Could you check a few things on this model? Use its own coordinates, in mm. A direction names the side the tool comes from. Round coordinates to 2 decimals unless told otherwise and drop trailing zeros. Loops run counter-clockwise (first coordinate to the right, second up) from the corner with the lowest first, then second, coordinate; pieces in that order, holes last. Notation, with made-up numbers: (-37.5, 51.5) -> (5.5, 51.5) arc R16 cw to (5.5, 73.5) -> close; hole circle Ø3 at (38, 48.5). An arc over 180 degrees is marked (long way). Write each question's results on one line, items separated by ' | '. Start each with the question number.
1) We'd pull the mould along Y, two halves only. Please class faces 1 (the flat face through (0, 3, 0)), 2 (the cylindrical face through (-0.33, -7.493, 3.944)), 3 (the flat face through (1.97, -3.48, 5.54)): pulls with the +Y half, pulls with the -Y half, needs draft (parallel to the pull), parting line crosses it, or undercut.
2) Imagine slicing it at C-C, the plane x = 1. List the corners of the cut face in (y, z) for me.
3) Imagine slicing it at A-A, the plane y = 0. List the corners of the cut face in (x, z) for me, plus the area to 3 significant figures.
4) Imagine slicing it at B-B, the plane z = 4.5. List the corners of the cut face in (x, y) for me, plus the area to 3 significant figures.
5) If I drill on probe 1 along X at (y, z) = (0, 0.7); probe 2 along X at (y, z) = (-3.5, 6.5), over which ranges is the centre line in solid material (lowest first)?
6) Imagine slicing it at D-D, the plane x = -3.75. List the corners of the cut face in (y, z) for me.
7) For P1, Ø2.5, axis at x = 0, y = -2, coming from the +Z side; P2, Ø3, axis at x = -3, z = 4, coming from the +Y side; P3, Ø1.5, axis at y = -4.5, z = 1, coming from the -X side, each with a flat end and sliding along its axis, tell me the tip position at first contact or that it passes through.
8) Which directions (+Z, -Z, +X, -X, +Y, -Y) give clear straight access to the entire face, cutting with the end or side of a thin tool? Please do faces 4 (the flat face through (3.2, 3.2, 8)), 5 (the flat face through (-1.97, 3.48, 5.54)).
from build123d import *

# Parameters (mm, degrees)
EXTRUDE001_DEPTH = 5
FACE_R           = 7.5
FACE_R_2         = 2.55
EXTRUDE_DEPTH    = 8


with BuildPart() as extrude001:
    # Sketch001 (on Face4 of Extrude) → Extrude001 (new body)
    with BuildSketch(Plane.XY.offset(8)):
        Polygon((4, -2.309401), (4, 2.309401), (0, 4.618802), (-4, 2.309401), (-4, -2.309401), (0, -4.618802), align=None)
    extrude(amount=-EXTRUDE001_DEPTH)


with BuildPart() as cut:
    # Face → Extrude (new body)
    with BuildSketch(Plane(origin=(0, 0, 0), x_dir=(0, 1, 0), z_dir=(0, 0, 1))):
        Circle(FACE_R)
        Circle(FACE_R_2, mode=Mode.SUBTRACT)
    extrude(amount=EXTRUDE_DEPTH)

    # Cut: cut Extrude001
    add(extrude001.part, mode=Mode.SUBTRACT)


solid = cut.part
Checked values:
1) face 1: needs draft | face 2: parting line crosses it | face 3: undercut
2) outline: (-7.43, 0) -> (-2.35, 0) -> (-2.35, 3) -> (-4.04, 3) -> (-4.04, 8) -> (-7.43, 8) -> close; (2.35, 0) -> (7.43, 0) -> (7.43, 8) -> (4.04, 8) -> (4.04, 3) -> (2.35, 3) -> close
3) outline: (-7.5, 0) -> (-2.55, 0) -> (-2.55, 3) -> (-4, 3) -> (-4, 8) -> (-7.5, 8) -> close; (2.55, 0) -> (7.5, 0) -> (7.5, 8) -> (4, 8) -> (4, 3) -> (2.55, 3) -> close | area: 64.7 mm^2
4) outline: circle Ø15 at (0, 0); hole (-4, -2.31) -> (0, -4.62) -> (4, -2.31) -> (4, 2.31) -> (0, 4.62) -> (-4, 2.31) -> close | area: 121 mm^2
5) probe 1: -7.5 to -2.55, 2.55 to 7.5 | probe 2: -6.63 to -1.94, 1.94 to 6.63
6) outline: (-6.5, 0) -> (6.5, 0) -> (6.5, 8) -> (2.45, 8) -> (2.45, 3) -> (-2.45, 3) -> (-2.45, 8) -> (-6.5, 8) -> close
7) P1: z = 3 | P2: y = 7.35 | P3: x = -6.5
8) face 4: +Z, +X, -X, +Y, -Y | face 5: +Z
